from build123d import *

# Parameters (mm, degrees)
IZIM1_W                     = 180
IZIM1_H                     = 56
IZIM1_W_2                   = 10
IZIM1_H_2                   = 6.5
Y_KSEKLIK_EKSTR_ZYON1_DEPTH = 5


with BuildPart() as part:
    # Çizim1 → Yükseklik-Ekstrüzyon1 (new body)
    with BuildSketch(Plane(origin=(0, 0, 0), x_dir=(1, 0, 0), z_dir=(0, 1, 0))):
        Rectangle(IZIM1_W, IZIM1_H)
        with Locations((-51.44343362, 20.75)):
            Rectangle(IZIM1_W_2, IZIM1_H_2, mode=Mode.SUBTRACT)
    extrude(amount=Y_KSEKLIK_EKSTR_ZYON1_DEPTH)


solid = part.part
Design review of the part built by this model. Coordinates are the model's own, in mm. A direction names the side the tool comes from. Coordinates: 2 decimals unless noted, no trailing zeros. Write each loop counter-clockwise with the first axis right and the second up, starting at its lowest first coordinate (ties: lowest second). Pieces come first, ordered by that corner, then holes. Notation, with made-up numbers: (-22.5, -12.75) -> (36.5, -12.75) arc R10 cw to (36.5, 5.25) -> close; hole circle Ø3 at (57.5, 70.5). An arc over 180 degrees is marked (long way). Write each question's results on one line, items separated by ' | '. Start each with the question number.
(1) For line 1 along X through (y, z) = (3.8, -20.5); line 2 along Z through (x, y) = (-48, 4.85), list the stretches that pass through material, from the lowest coordinate up. Write a range as from..to.
(2) Clearance check with a flat-ended pin moving along its axis: P1, Ø4, axis at x = -9, z = -0.5, coming from the -Y side. State where the tip first meets the part, or that it passes through.
(3) Take a section at B-B on x = -49.5. Write out the cut boundary in (y, z), and give its area (4 significant figures).
(4) Tool access review of faces 1 (the face through (-1, 5, 0)), 2 (the face through (-52, 2, -17.5)): name each direction out of +Z, -Z, +X, -X, +Y, -Y from which nothing blocks a thin tool from reaching the whole face with its end or side.
(5) Take a section at A-A on z = -21.5. Write out the cut boundary in (x, y).
(6) The part is to be moulded in two halves that separate along Z. For faces 3 (the face through (90, 2, 0)), 4 (the face through (-56.443, 2, -21)), 5 (the face through (-1, 2, -28)), say which applies: pulls with the +Z half, pulls with the -Z half, needs draft (parallel to the pull), parting line crosses it, or undercut.
Results found:
1) line 1: x = -90..-56.44, -46.44..90 | line 2: z = -28..-24, -17.5..28
2) P1: stops at y = 0
3) outline: (0, -28) -> (5, -28) -> (5, -24) -> (0, -24) -> close; (0, -17.5) -> (5, -17.5) -> (5, 28) -> (0, 28) -> close | area: 247.5 mm2
4) face 1: +Z, -Z, +X, -X, +Y | face 2: +Y, -Y
5) outline: (-90, 0) -> (-56.44, 0) -> (-56.44, 5) -> (-90, 5) -> close; (-46.44, 0) -> (90, 0) -> (90, 5) -> (-46.44, 5) -> close
6) face 3: needs draft | face 4: undercut | face 5: pulls with the -Z half
